Print and shaded views of the part. All mm, measured from the part's lowest x, y and z. A direction names the side the tool comes from. Round coordinates to 2 decimals unless told otherwise and drop trailing zeros. Write each loop counter-clockwise with the first axis right and the second up, starting at its lowest first coordinate (ties: lowest second). Pieces come first, ordered by that corner, then holes. Notation, with made-up numbers: (23, 53) - (43, 53) arc R21 cw to (43, 83) - close; hole circle Ø6 at (18, 3). An arc over 180 degrees is marked (long way). One line per item, written item: value.
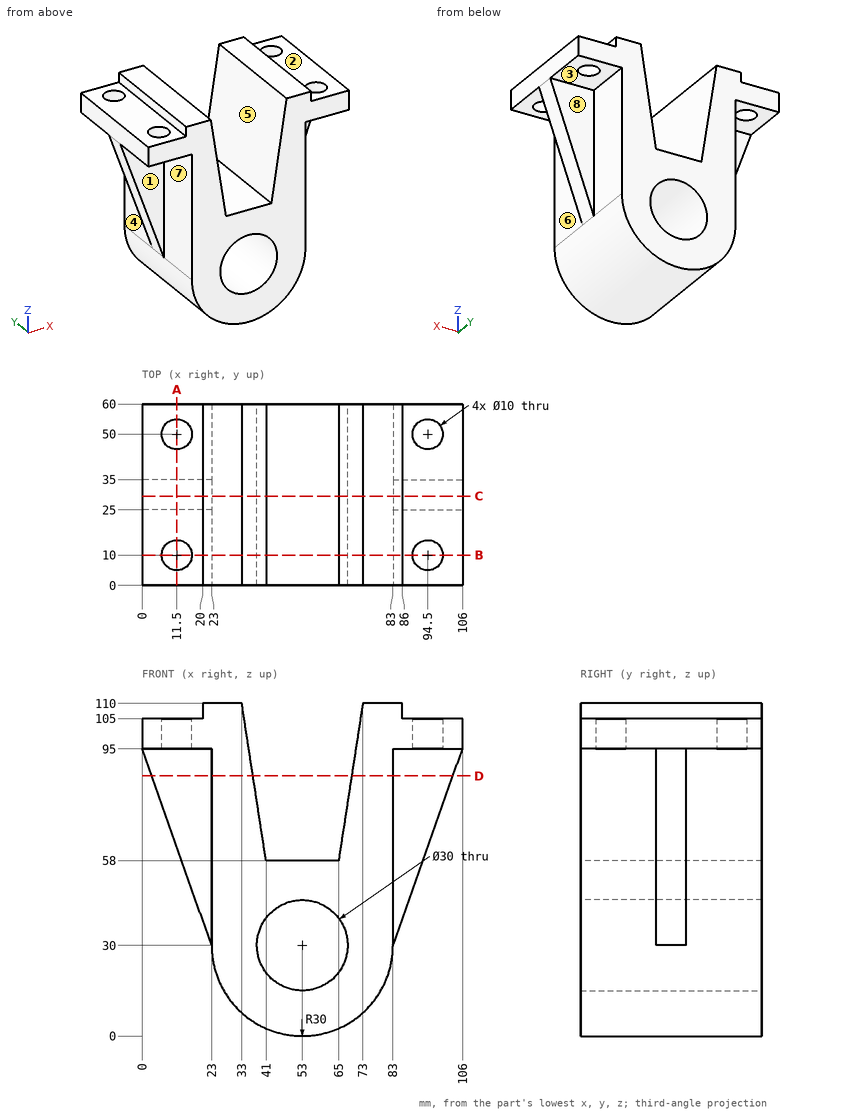
1. Band-saw the part on A-A on x = 11.5. Write the cut outline in (y, z), plus the area to 3 significant figures.
Report:
outline: (0, 95) - (5, 95) - (5, 105) - (0, 105) - close; (15, 95) - (25, 95) - (25, 62.5) - (35, 62.5) - (35, 95) - (45, 95) - (45, 105) - (15, 105) - close; (55, 95) - (60, 95) - (60, 105) - (55, 105) - close
area: 725 mm²
2. Band-saw the part on C-C on y = 29.5. Write the cut outline in (x, z).
Report:
outline: (0, 95) - (23, 30) arc R30 ccw to (83, 30) - (106, 95) - (106, 105) - (86, 105) - (86, 110) - (73, 110) - (65, 58) - (41, 58) - (33, 110) - (20, 110) - (20, 105) - (0, 105) - close; hole circle Ø30 at (53, 30)
3. Mould opens along X. For the marked faces 5, 6, 7 and 8 say: released by +X, released by -X, zero draft, split by the parting line, or undercut.
Report:
face 5: undercut
face 6: released by +X
face 7: released by -X
face 8: zero draft
4. Drop flat-ended pins along their axis: pin 1 (1.5 mm diameter, centred on x = 90.5, y = 36.5, fed in from -Z); pin 2 (1 mm diameter, centred on y = 34, z = 38, fed in from +X); pin 3 (10 mm diameter, centred on y = 47.5, z = 54, fed in from +X). Give the stop position or say it passes through.
Report:
pin 1: z = 95
pin 2: x = 86.01
pin 3: x = 83
5. Wall check: probe 1 along Y at (x, z) = (94.5, 97.5); probe 2 along X at (y, z) = (8.5, 39); probe 3 along X at (y, z) = (55, 23). Give the ranges that are in metal, low to high. Write a range as [from, to].
Report:
probe 1: [0, 5], [15, 45], [55, 60]
probe 2: [23, 41], [65, 83]
probe 3: [23.83, 39.73], [66.27, 82.17]
6. Tool access for the marked faces 1, 2, 3 and 4: list every direction of +Z, -Z, +X, -X, +Y, -Y with a clear straight run to the whole face (end or side of a thin tool).
Report:
face 1: -Z, -X, -Y
face 2: +Z, +X, +Y, -Y
face 3: -Z, +X, +Y
face 4: -Z, -X, +Y
7. Band-saw the part on D-D on z = 86. Write the cut outline in (x, y).
Report:
outline: (3.18, 25) - (23, 25) - (23, 0) - (36.69, 0) - (36.69, 60) - (23, 60) - (23, 35) - (3.18, 35) - close; (69.31, 0) - (83, 0) - (83, 25) - (102.82, 25) - (102.82, 35) - (83, 35) - (83, 60) - (69.31, 60) - close
8. Band-saw the part on B-B on y = 10. Write the cut outline in (x, z).
Report:
outline: (0, 95) - (6.5, 95) - (6.5, 105) - (0, 105) - close; (16.5, 95) - (23, 95) - (23, 30) arc R30 ccw to (83, 30) - (83, 95) - (89.5, 95) - (89.5, 105) - (86, 105) - (86, 110) - (73, 110) - (65, 58) - (41, 58) - (33, 110) - (20, 110) - (20, 105) - (16.5, 105) - close; (99.5, 95) - (106, 95) - (106, 105) - (99.5, 105) - close; hole circle Ø30 at (53, 30)
